Design review of the part built by this model. Coordinates are the model's own, in mm. A direction names the side the tool comes from. Give positions to 0.01 mm unless a question says otherwise; leave off trailing zeros. Loops run counter-clockwise (first coordinate to the right, second up) from the corner with the lowest first, then second, coordinate; pieces in that order, holes last. Notation, with made-up numbers: M -29,-40 L -16,-40 A12 ccw -16,-33 Z; hole C -25.5,76 d6. An arc over 180 degrees is marked long. Answer as CSV lines item,"result".
Autodesk Inventor part; units mm, degrees
ref_plane "YZ Plane" through (0, 0, 0) normal (1, 0, 0) x (0, 1, 0)
ref_plane "XZ Plane" through (0, 0, 0) normal (0, 1, 0) x (-1, 0, 0)
ref_plane "XY Plane" through (0, 0, 0) normal (0, 0, 1) x (1, 0, 0)
sketch "Sketch1" plane through (0, 0, 0) normal (0, 1, 0) x (-1, 0, 0)
  line L0 (0, 0) -> (-152.4, 0)
  line L1 (-152.4, 0) -> (-152.4, 76.2)
  line L2 (-152.4, 76.2) -> (0, 76.2)
  line L3 (0, 76.2) -> (0, 0)
extrude "Extrusion1" add sketch "Sketch1" along normal blind 3.175
sketch "Sketch2" plane through (0, 3.175, 0) normal (0, 1, 0) x (1, 0, 0)
  point P0 (0, 0)
sketch "Sketch3" plane through (0, 3.175, 0) normal (0, 1, 0) x (1, 0, 0)
  point P0 (0, 0)
sketch "Sketch4" plane through (0, 3.175, 0) normal (0, 1, 0) x (1, 0, 0)
  circle A0 centre (6.35, -6.35) radius 3.175
  circle A1 centre (6.35, -69.9426) radius 3.175
  circle A2 centre (145.8663, -69.9426) radius 3.175
  circle A3 centre (145.8663, -6.35) radius 3.175
  point P0 (0, 0)
hole "Hole1" at (6.35, 3.175, 6.35) at (6.35, 3.175, 69.9426) at (145.8663, 3.175, 69.9426) at (145.8663, 3.175, 6.35) direction (0, -1, 0) diameter 6.35 end through all
sketch "Sketch5" plane through (0, 3.175, 0) normal (0, 1, 0) x (1, 0, 0)
  line L0 (10.5157, -11.0499) -> (10.5124, -63.5081)
  arc A0 (16.7318, -11.0499) -> (10.5157, -11.0499) centre (13.6238, -10.7421) ccw
  arc A1 (10.5124, -63.5081) -> (16.7351, -63.5081) centre (13.6238, -63.5083) ccw
  line L1 (16.7318, -24.057) -> (34.8293, -8.3141)
  line L2 (16.7369, -34.4606) -> (39.8985, -14.1414)
  line L3 (16.7369, -34.4606) -> (39.3705, -61.398)
  line L4 (34.3364, -65.6278) -> (16.7351, -44.6796)
  line L5 (16.7318, -11.0499) -> (16.7318, -24.057)
  line L6 (16.7351, -44.6796) -> (16.7351, -63.5081)
  arc A2 (39.8985, -14.1414) -> (34.8293, -8.3141) centre (37.3639, -11.2278) ccw
  arc A3 (34.3364, -65.6278) -> (39.3705, -61.398) centre (36.8535, -63.5129) ccw
  arc A4 (61.8542, -17.5534) -> (61.8542, -11.2278) centre (61.8542, -14.3906) ccw
  arc A5 (61.8927, -39.7278) -> (61.8542, -33.4021) centre (61.8734, -36.5649) ccw
  arc A6 (61.8542, -63.5501) -> (61.8542, -57.2244) centre (61.8542, -60.3873) ccw
  line L7 (61.8542, -11.2278) -> (47.9378, -11.2278)
  line L8 (49.1549, -33.4021) -> (49.1549, -17.5534)
  line L9 (49.1549, -39.7278) -> (49.1549, -57.2244)
  line L10 (61.8542, -57.2244) -> (49.1549, -57.2244)
  line L11 (61.8927, -39.7278) -> (49.1549, -39.7278)
  line L12 (61.8542, -17.5534) -> (49.1549, -17.5534)
  line L13 (49.1549, -33.4021) -> (61.8542, -33.4021)
  arc A7 (47.9378, -11.2278) -> (41.5878, -16.1855) centre (47.2856, -16.9379) ccw
  line L14 (41.5878, -16.1855) -> (41.5878, -57.5593)
  line L15 (49.1549, -63.5501) -> (61.8542, -63.5501)
  arc A8 (41.5878, -57.5593) -> (49.1549, -63.5501) centre (49.1549, -55.7757) ccw
  line L16 (67.0028, -13.2236) -> (76.6357, -60.4074)
  line L17 (93.2217, -13.986) -> (81.9862, -60.5027)
  line L18 (73.3373, -13.1484) -> (79.3224, -40.4995)
  line L19 (79.3224, -40.4995) -> (87.3283, -12.4343)
  arc A9 (73.3373, -13.1484) -> (67.0028, -13.2236) centre (70.1778, -13.8398) ccw
  arc A10 (93.2217, -13.986) -> (87.3283, -12.4343) centre (90.2592, -13.2704) ccw
  arc A11 (76.6357, -60.4074) -> (81.9862, -60.5027) centre (79.3216, -59.8591) ccw
  circle A12 centre (100.2447, -14.3906) radius 3.175
  line L20 (97.0697, -32.199) -> (97.0697, -60.5027)
  line L21 (103.4197, -32.199) -> (103.4197, -60.5027)
  arc A13 (97.0697, -60.5027) -> (103.4197, -60.5027) centre (100.2447, -60.5027) ccw
  arc A14 (103.4197, -32.199) -> (97.0697, -32.199) centre (100.2447, -32.199) ccw
  line L22 (109.3457, -13.3836) -> (109.3457, -60.5027)
  line L23 (141.7333, -14.3906) -> (141.7333, -60.5027)
  arc A15 (109.3457, -60.5027) -> (115.6957, -60.5027) centre (112.5207, -60.5027) ccw
  arc A16 (115.6957, -13.3836) -> (109.3457, -13.3836) centre (112.5207, -13.3836) ccw
  arc A17 (141.7333, -14.3906) -> (135.3833, -14.3906) centre (138.5583, -14.3906) ccw
  arc A18 (135.3833, -60.5027) -> (141.7333, -60.5027) centre (138.5583, -60.5027) ccw
  line L24 (115.6957, -17.5656) -> (135.3833, -41.317)
  line L25 (115.6957, -32.199) -> (135.3833, -55.7757)
  line L26 (135.3833, -14.3906) -> (135.3833, -41.317)
  line L27 (135.3833, -55.7757) -> (135.3833, -60.5027)
  line L28 (115.6957, -32.199) -> (115.6957, -60.5027)
  line L29 (115.6957, -17.5656) -> (115.6957, -13.3836)
  point P0 (0, 0)
sketch "Sketch6" plane through (0, 3.175, 0) normal (0, 1, 0) x (1, 0, 0)
  point P0 (0, 0)
extrude "Extrusion2" cut sketch "Sketch5" against normal blind 2.54
properties part number "klam final"
1. For faces 4 (the flat face through (100, 0.635, 14)), 5 (the flat face through (77, 0, 39)), list the 3-axis set-ups (+Z, -Z, +X, -X, +Y, -Y) from which the entire face can be reached by the end or side of a thin tool; tool diameter is ignored.
Answer block:
face 4,"+Y"
face 5,"+Z, -Z, +X, -X, -Y"
2. The part is to be moulded in two halves that separate along Z. For faces 1 (the cylindrical face through (148.966, 1.565, 69.254)), 2 (the flat face through (77, 2, 76.2)), 3 (the flat face through (152.4, 2, 38)), say which applies: pulls with the +Z half, pulls with the -Z half, needs draft (parallel to the pull), parting line crosses it, or undercut.
Answer block:
face 1,"undercut"
face 2,"pulls with the +Z half"
face 3,"needs draft"
3. For P1, Ø3, axis at x = 48.5, z = 39, coming from the +Y side (3 decimals); P2, Ø5, axis at x = 13.62, z = 10.74, coming from the +Y side (3 decimals), all flat-tipped, find the tip position at first contact; note any pin that passes through.
Answer block:
P1,"y = 3.175"
P2,"y = 0.635"
4. We need section D-D, the plane y = 1.9. Count the separate pieces of the cut face and the enclosed holes in it, plus the area to 3 significant figures.
Answer block:
separate pieces,"1"
enclosed holes,"10"
area,"8,220 mm²"
5. We need section B-B, the plane x = 60. Write out the cut boundary in (y, z) (3 decimals).
Answer block:
outline,"M 0,0 L 3.175,0 L 3.175,11.228 L 0.635,11.228 L 0.635,17.553 L 3.175,17.553 L 3.175,33.402 L 0.635,33.402 L 0.635,39.728 L 3.175,39.728 L 3.175,57.224 L 0.635,57.224 L 0.635,63.55 L 3.175,63.55 L 3.175,76.2 L 0,76.2 Z"
6. We need section A-A, the plane x = 6.35. Write out the cut boundary in (y, z) (3 decimals).
Answer block:
outline,"M 0,0 L 3.175,0 L 3.175,3.175 L 0,3.175 Z; M 0,9.525 L 3.175,9.525 L 3.175,66.768 L 0,66.768 Z; M 0,73.118 L 3.175,73.118 L 3.175,76.2 L 0,76.2 Z"
7. To check wall thickness, follow L1, parallel to X at y = 0.9, z = 6.35 (3 decimals); L2, parallel to Z at x = 54, y = 1.45; L3, parallel to X at y = 1.6, z = 11. State the ranges of each line that lie inside material, in increasing order. Write a range as [from, to].
Answer block:
L1,"[0, 3.175], [9.525, 142.691], [149.041, 152.4]"
L2,"[0, 11.23], [17.55, 33.4], [39.73, 57.22], [63.55, 76.2]"
L3,"[0, 10.51], [16.74, 31.74], [41.22, 68.63], [71.73, 88.23], [92.29, 110.42], [114.62, 152.4]"
